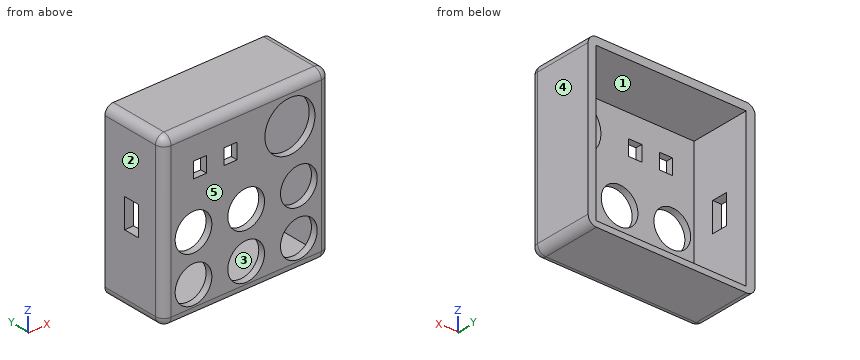
from build123d import *

# Parameters (mm, degrees)
F0_W      = 100
F0_H      = 100
F0_R      = 11
F0_R_2    = 15
F1_DEPTH  = 40
F2_W      = 89.999996
F2_H      = 92
F3_DEPTH  = 36
F4_W      = 7.8
F4_H      = 9.3
F5_DEPTH  = 25
F6_R      = 5
F7_R      = 5
F8_R      = 5
F9_W      = 9.469847
F9_H      = 17.487352
F10_DEPTH = 25


with BuildPart() as f1:
    # F0 (on Front) → F1 (new body)
    with BuildSketch(Plane.XZ):
        Rectangle(F0_W, F0_H)
        with Locations((-31.548171, -32.950651)):
            Circle(F0_R, mode=Mode.SUBTRACT)
        with Locations((-31.548173, -5.504166)):
            Circle(F0_R, mode=Mode.SUBTRACT)
        with Locations((-3e-06, -5.504166)):
            Circle(F0_R, mode=Mode.SUBTRACT)
        with Locations((0, -32.950651)):
            Circle(F0_R, mode=Mode.SUBTRACT)
        with Locations((31.548171, -32.950651)):
            Circle(F0_R, mode=Mode.SUBTRACT)
        with Locations((31.548168, -5.504166)):
            Circle(F0_R, mode=Mode.SUBTRACT)
        with Locations((26.192216, 27.900403)):
            Circle(F0_R_2, mode=Mode.SUBTRACT)
    extrude(amount=F1_DEPTH)

    # F2 (on face) → F3 (cut)
    with BuildSketch(Plane(origin=(0, 0, 0), x_dir=(-1, 0, 0), z_dir=(0, 1, 0))):
        with Locations((-0.403937, -0.61572)):
            Rectangle(F2_W, F2_H)
    extrude(amount=-F3_DEPTH, mode=Mode.SUBTRACT)

    # F4 (on face) → F5 (cut)
    with BuildSketch(Plane.XZ.offset(40)):
        with Locations((-9.38255, 27.058275)):
            Rectangle(F4_W, F4_H)
        with Locations((-27.672551, 27.058275)):
            Rectangle(F4_W, F4_H)
    extrude(amount=-F5_DEPTH, mode=Mode.SUBTRACT)

    # F6
    f6_edges = [f1.edges().sort_by_distance(p)[0] for p in [
        (50, -40, 0),
    ]]
    fillet(f6_edges, radius=F6_R)

    # F7
    f7_edges = [f1.edges().sort_by_distance(p)[0] for p in [
        (-50, -40, 0),
    ]]
    fillet(f7_edges, radius=F7_R)

    # F8
    f8_edges = [f1.edges().sort_by_distance(p)[0] for p in [
        (0, -40, -50),
        (0, -40, 50),
    ]]
    fillet(f8_edges, radius=F8_R)

    # F9 (on face) → F10 (cut)
    with BuildSketch(Plane(origin=(-50, 0, 0), x_dir=(0, -1, 0), z_dir=(-1, 0, 0))):
        with Locations((18.386893, -0.142781)):
            Rectangle(F9_W, F9_H)
    extrude(amount=-F10_DEPTH, mode=Mode.SUBTRACT)


solid = f1.part
The model under review builds one solid part; all positions refer to its coordinate system, in mm. Face numbers are marked on the shaded views. A direction names the side the tool comes from. Give positions to 0.01 mm unless a question says otherwise; leave off trailing zeros. Write each loop counter-clockwise with the first axis right and the second up, starting at its lowest first coordinate (ties: lowest second). Pieces come first, ordered by that corner, then holes.
1. Add section D-D, the plane z = 37.5. Write out the cut boundary in (x, y), plus the area to 3 significant figures.
2. Add section B-B, the plane y = -7.5. Write out the cut boundary in (x, z), plus the area to 3 significant figures.
3. For P1, Ø1.2, axis at y = -39, z = 25, coming from the +X side; P2, Ø8, axis at x = 1, z = -27, coming from the +Y side; P3, Ø8, axis at x = 17, z = -32, coming from the +Y side; P4, Ø1.2, axis at x = -9, y = -37, coming from the +Z side, all flat-tipped, find the tip position at first contact; note any pin that passes through.
4. Draft analysis for pull direction X (two halves, no side actions). For the marked faces 3, 4 and 5, state which applies: +X half, -X half, draft (parallel to the pull), parting line (faces both ways), or undercut.
5. Tool access review of the marked faces 1 and 2: name each direction out of +Z, -Z, +X, -X, +Y, -Y from which nothing blocks a thin tool from reaching the whole face with its end or side.
6. Add section A-A, the plane x = 0. Write out the cut boundary in (y, z), plus the area to 3 significant figures.
7. Add section C-C, the plane z = 26.5. Write out the cut boundary in (x, y).
8. Wall thickness on L1, parallel to Z at x = -42, y = -6; L2, parallel to X at y = -10.5, z = -6.5; L3, parallel to Z at x = 0, y = -37: over which ranges is each line inside the solid? List them lowest first.
Worked answers:
1. outline: (-50, -35) arc R5 ccw to (-45, -40) - (14.67, -40) - (14.67, -36) - (-44.6, -36) - (-44.6, 0) - (-50, 0) - close; (37.72, -40) - (45, -40) arc R5 ccw to (50, -35) - (50, 0) - (45.4, 0) - (45.4, -36) - (37.72, -36) - close
1. area: 657 mm2
2. outline: (-50, -45) arc R5 ccw to (-45, -50) - (45, -50) arc R5 ccw to (50, -45) - (50, 45) arc R5 ccw to (45, 50) - (-45, 50) arc R5 ccw to (-50, 45) - close; hole (-44.6, -46.62) - (45.4, -46.62) - (45.4, 45.38) - (-44.6, 45.38) - close
2. area: 1,700 mm2
3. P1: stops at x = 48.67
3. P2: passes through
3. P3: stops at y = -36
3. P4: stops at z = 49.8
4. face 3: undercut
4. face 4: +X half
4. face 5: draft
5. face 1: +Y
5. face 2: +Z, -Z, -X, +Y, -Y
6. outline: (-40, -45) arc R5 ccw to (-35, -50) - (0, -50) - (0, -46.62) - (-36, -46.62) - (-36, -43.95) - (-40, -43.95) - close; (-40, -21.95) - (-36, -21.95) - (-36, -16.5) - (-40, -16.5) - close; (-40, 5.5) - (-36, 5.5) - (-36, 45.38) - (0, 45.38) - (0, 50) - (-35, 50) arc R5 ccw to (-40, 45) - close
6. area: 501 mm2
7. outline: (-50, -35) arc R5 ccw to (-45, -40) - (-31.57, -40) - (-31.57, -36) - (-44.6, -36) - (-44.6, 0) - (-50, 0) - close; (-23.77, -40) - (-13.28, -40) - (-13.28, -36) - (-23.77, -36) - close; (-5.48, -40) - (11.26, -40) - (11.26, -36) - (-5.48, -36) - close; (41.13, -40) - (45, -40) arc R5 ccw to (50, -35) - (50, 0) - (45.4, 0) - (45.4, -36) - (41.13, -36) - close
8. L1: z = -50 to -46.62, 45.38 to 50
8. L2: x = -50 to -44.6, 45.4 to 50
8. L3: z = -49.58 to -43.95, -21.95 to -16.5, 5.5 to 49.58
